Input: part model. Units: mm. Frame: model coordinates. Face numbers are marked on the shaded views. A direction names the side the tool comes from. Coordinates: 2 decimals unless noted, no trailing zeros. Write each loop counter-clockwise with the first axis right and the second up, starting at its lowest first coordinate (ties: lowest second). Pieces come first, ordered by that corner, then holes. Notation, with made-up numbers: (-33, 65) -> (-18, 65) arc R11 cw to (-18, 71) -> close; hole circle Ø11 at (21, 66). An arc over 180 degrees is marked (long way). Use one line per item in the form item = value. Start each with the question number.
(1) First-contact query: pin 1 (2.5 mm diameter, centred on y = 0, z = 0, fed in from -X); pin 2 (1.5 mm diameter, centred on x = -3, y = 2.5, fed in from -Z). Flat tips, straight axial feed; report the tip coordinate or a pass-through.
(2) Cut plane A-A on y = 0. Return the cut outline in (x, z).
(3) Ray query, line 1 along Z through (x, y) = (-1.25, 0); line 2 along X through (y, z) = (-1, -3.5). Return the intervals inside material, ascending.
(4) Pull-direction query (Z, two-part tool) for the marked faces 3, 4 and 5; classes: released by +Z, released by -Z, zero draft, split by the parting line, or undercut.
(5) Set-up query: the marked faces 1 and 2. Return all of +Z, -Z, +X, -X, +Y, -Y with unobstructed straight access to the full face (end or side cutting, diameter ignored); none if empty.
(6) Cut plane D-D on y = -3.5. Return the cut outline in (x, z).
(7) Cut plane B-B on z = 0. Return the cut outline in (x, y), plus the area to 3 significant figures.
(8) Cut plane C-C on x = -2.5. Return the cut outline in (y, z).
Autodesk Inventor part; units mm, degrees
ref_plane "nut_XY" through (0, 0, 0) normal (1, 0, 0) x (0, 0, -1)
ref_plane "nut_YZ" through (0, 0, 0) normal (0, 0, -1) x (0, 1, 0)
ref_plane "nut_ZX" through (0, 0, 0) normal (0, 1, 0) x (1, 0, 0)
sketch "Sketch_1" plane through (0, 0, 0) normal (0, 0, 1) x (1, 0, 0)
  line L0 (-2, -4) -> (-1, -5)
  line L1 (-1, -5) -> (0, -5)
  line L2 (0, -5) -> (0, 5)
  line L3 (0, 5) -> (-1, 5)
  line L4 (-1, 5) -> (-2, 4)
  line L5 (-2, 4) -> (-2, -4)
extrude "Extrusion1" add sketch "Sketch_1" along normal mid plane 10
sketch "Sketch_10" plane through (0, 0, 0) normal (0, 0, 1) x (1, 0, 0)
  line L0 (-2, 0) -> (-3.7, 0)
  line L1 (-3.7, 0) -> (-3.7, 3)
  line L2 (-3.7, 3) -> (-2, 3.35)
  line L3 (-2, 3.35) -> (-2, 0)
  line L4 (-2, 0) -> (-3.7, 0)
revolve "Revolution1" add sketch "Sketch_10" angle 360 about axis through (-2, 0, 0) along (1, 0, 0)
sketch "Sketch_3" plane through (0, 0, 0) normal (0, 0, 1) x (1, 0, 0)
  line L0 (0, 0) -> (-3.7, 0)
  line L1 (-3.7, 0) -> (-3.7, 2.5)
  line L2 (-3.7, 2.5) -> (-3.267, 2.067)
  line L3 (-3.267, 2.067) -> (-0.433, 2.067)
  line L4 (-0.433, 2.067) -> (0, 2.5)
  line L5 (0, 2.5) -> (0, 0)
  line L6 (0, 0) -> (-3.7, 0)
revolve "Revolution2" cut sketch "Sketch_3" angle 360 about axis through (0, 0, 0) along (1, 0, 0)
thread "Thread1"
ref_plane "nut_XY" through (0, 0, 0) normal (1, 0, 0) x (0, 0, -1)
ref_plane "nut_YZ" through (0, 0, 0) normal (0, 0, -1) x (0, 1, 0)
ref_plane "nut_ZX" through (0, 0, 0) normal (0, 1, 0) x (1, 0, 0)
ref_plane "to_bolt_XY" through (-3.7, 0, 0) normal (1, 0, 0) x (0, 0, -1)
ref_plane "to_bolt_YZ" through (-3.7, 0, 0) normal (0, 0, -1) x (0, 1, 0)
ref_plane "to_bolt_ZX" through (-3.7, 0, 0) normal (0, 1, 0) x (1, 0, 0)
ref_plane "to_frames_XY" through (-2, 0, 0) normal (1, 0, 0) x (0, 0, -1)
ref_plane "to_frames_YZ" through (-2, 0, 0) normal (0, 0, -1) x (0, 1, 0)
ref_plane "to_frames_ZX" through (-2, 0, 0) normal (0, 1, 0) x (1, 0, 0)
properties part number "HNTTBS5-5"
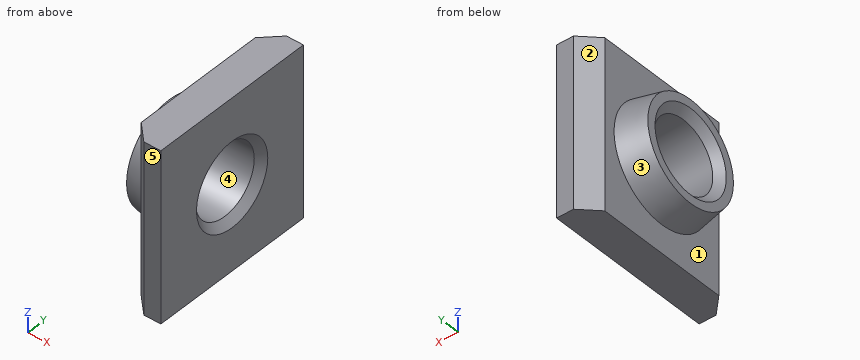
Values:
q1.pin_1 = through
q1.pin_2 = -2.65
q2.outline = (-3.7, -3) -> (-2, -3.35) -> (-2, -5) -> (0, -5) -> (0, -2.5) -> (-0.43, -2.07) -> (-3.27, -2.07) -> (-3.7, -2.5) -> close; (-3.7, 2.5) -> (-3.27, 2.07) -> (-0.43, 2.07) -> (0, 2.5) -> (0, 5) -> (-2, 5) -> (-2, 3.35) -> (-3.7, 3) -> close
q3.line_1 = -5 to -2.07, 2.07 to 5
q3.line_2 = -2 to 0
q4.face_3 = split by the parting line
q4.face_4 = undercut
q4.face_5 = zero draft
q5.face_1 = -X
q5.face_2 = +Z, -Z, -X, +Y
q6.outline = (-2, -5) -> (0, -5) -> (0, 5) -> (-2, 5) -> close
q7.outline = (-3.7, -3) -> (-2, -3.35) -> (-2, -4) -> (-1, -5) -> (0, -5) -> (0, -2.5) -> (-0.43, -2.07) -> (-3.27, -2.07) -> (-3.7, -2.5) -> close; (-3.7, 2.5) -> (-3.27, 2.07) -> (-0.43, 2.07) -> (0, 2.5) -> (0, 5) -> (-1, 5) -> (-2, 4) -> (-2, 3.35) -> (-3.7, 3) -> close
q7.area = 14.1 mm2
q8.outline = circle Ø6.49 at (0, 0); hole circle Ø4.13 at (0, 0)
